Could you check a few things on this drawing? It's one solid part, dimensions in mm from its lowest x, y, z. Give positions to 0.01 mm unless a question says otherwise; leave off trailing zeros. Order: outer loops, then holes, each group sorted by start corner. A loop starts at its lowest first (then second) coordinate and runs counter-clockwise, first axis right, second up. Notation, with made-up numbers: (20, 75) - (70, 75) arc R12 cw to (70, 95) - close; hole circle Ø7 at (31.5, 3). An arc over 180 degrees is marked (long way). Return JSON: item names as keys, results as strings.
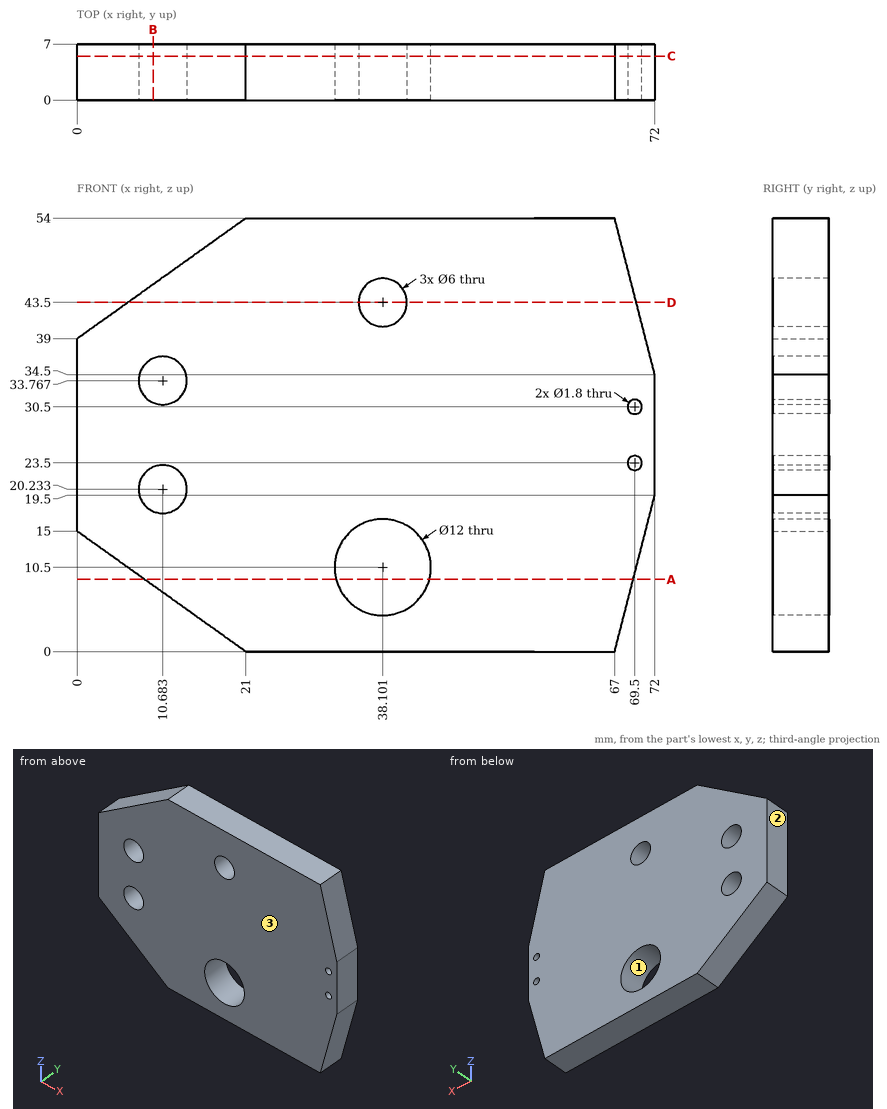
1. Thinking about a two-plate mould opening in X: for the marked faces 1, 2 and 3, which applies, +X half, -X half, draft (parallel to the pull), parting line (faces both ways), or undercut?
Checks:
{"face 1": "undercut", "face 2": "-X half", "face 3": "draft"}
2. Suppose I cut it at B-B (x = 9.5). List the corners of the cut face in (y, z) for me.
Checks:
{"outline": "(0, 8.21) - (7, 8.21) - (7, 17.48) - (0, 17.48) - close; (0, 22.99) - (7, 22.99) - (7, 31.01) - (0, 31.01) - close; (0, 36.52) - (7, 36.52) - (7, 45.79) - (0, 45.79) - close"}
3. Suppose I cut it at D-D (z = 43.5). List the corners of the cut face in (x, y) for me, plus the area to 3 significant figures.
Checks:
{"outline": "(6.3, 0) - (35.1, 0) - (35.1, 7) - (6.3, 7) - close; (41.1, 0) - (69.69, 0) - (69.69, 7) - (41.1, 7) - close", "area": "402 mm^2"}
4. If I drill on L1, parallel to Z at x = 36, y = 5.75; L2, parallel to Z at x = 8, y = 5 (1 decimal); L3, parallel to X at y = 1.75, z = 30, over which ranges is the centre line in solid material (lowest first)? Write a range as [from, to].
Checks:
{"L1": "[0, 4.88], [16.12, 41.36], [45.64, 54]", "L2": "[9.3, 18.9], [21.6, 32.4], [35.1, 44.7]", "L3": "[0, 68.75], [70.25, 72]"}
5. Suppose I cut it at C-C (y = 5.5). List the corners of the cut face in (x, z) for me.
Checks:
{"outline": "(0, 15) - (21, 0) - (67, 0) - (72, 19.5) - (72, 34.5) - (67, 54) - (21, 54) - (0, 39) - close; hole circle Ø6 at (10.68, 20.23); hole circle Ø6 at (10.68, 33.77); hole circle Ø12 at (38.1, 10.5); hole circle Ø6 at (38.1, 43.5); hole circle Ø1.8 at (69.5, 23.5); hole circle Ø1.8 at (69.5, 30.5)"}
6. Suppose I cut it at A-A (z = 9). List the corners of the cut face in (x, y) for me, plus the area to 3 significant figures.
Checks:
{"outline": "(8.4, 0) - (32.29, 0) - (32.29, 7) - (8.4, 7) - close; (43.91, 0) - (69.31, 0) - (69.31, 7) - (43.91, 7) - close", "area": "345 mm^2"}
